```python
from build123d import *

# Parameters (mm, degrees)
F0_W     = 50
F0_H     = 25
F1_DEPTH = 3
F3_D     = 3.2
F4_D     = 3.2
F5_D     = 3.2
F6_D     = 3.2


with BuildPart() as f1:
    # F0 (on Top) → F1 (new body)
    with BuildSketch(Plane.XY):
        with Locations((25, 12.5)):
            Rectangle(F0_W, F0_H)
    extrude(amount=F1_DEPTH)

    # F3 (through all)
    with Locations(Plane.XY.offset(3)):
        with Locations((2.12132, 22.87868)):
            Hole(F3_D / 2)

    # F4 (through all)
    with Locations(Plane.XY.offset(3)):
        with Locations((2.12132, 2.12132)):
            Hole(F4_D / 2)

    # F5 (through all)
    with Locations(Plane.XY.offset(3)):
        with Locations((47.87868, 2.12132)):
            Hole(F5_D / 2)

    # F6 (through all)
    with Locations(Plane.XY.offset(3)):
        with Locations((47.87868, 22.87868)):
            Hole(F6_D / 2)


solid = f1.part
```
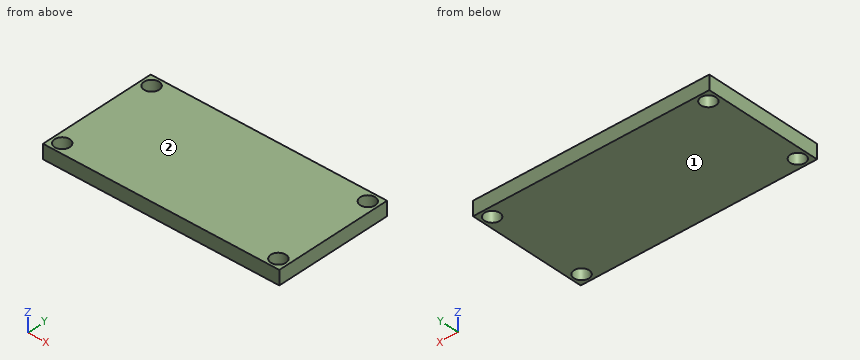
Geometry check sheet. Reference: the model listing, model coordinates, mm. Face numbers are marked on the shaded views. Coordinates: 2 decimals unless noted, no trailing zeros. Order: outer loops, then holes, each group sorted by start corner. A loop starts at its lowest first (then second) coordinate and runs counter-clockwise, first axis right, second up. Notation, with made-up numbers: (55, -11) - (68, -11) arc R22 cw to (68, -3) - close; hole circle Ø4 at (59, 10). An arc over 180 degrees is marked (long way). Answer in a Markdown table with one row per item. Add a question column.
1. Section check A-A (z = 0.6). Enter the section's corners in (x, y).
2. Gauge pin test, flat ends, axial feed: pin 1 Ø5 at (x, y) = (23, 11) entering from -Z; pin 2 Ø1.9 at (x, y) = (47.88, 2.12) entering from +Z. Record the tip position at first contact, or that the pin passes through.
3. Draft check along Z on the marked faces 1 and 2. Enter one of: +Z half, -Z half, draft (parallel to the pull), parting line (faces both ways), or undercut.
4. Material ranges on L1, parallel to X at y = 1.5, z = 2.6; L2, parallel to X at y = 2.5, z = 2.55, recorded low to high. Write a range as [from, to].
Data:
| question | item | result |
|---|---|---|
| 1 | outline | (0, 0) - (50, 0) - (50, 25) - (0, 25) - close; hole circle Ø3.2 at (2.12, 2.12); hole circle Ø3.2 at (2.12, 22.88); hole circle Ø3.2 at (47.88, 2.12); hole circle Ø3.2 at (47.88, 22.88) |
| 2 | pin 1 | stops at z = 0 |
| 2 | pin 2 | passes through |
| 3 | face 1 | -Z half |
| 3 | face 2 | +Z half |
| 4 | L1 | x = [0, 0.65], [3.6, 46.4], [49.35, 50] |
| 4 | L2 | x = [0, 0.57], [3.68, 46.32], [49.43, 50] |
